Could you check a few things on this model? Use its own coordinates, in mm. A direction names the side the tool comes from. Give positions to 0.01 mm unless a question says otherwise; leave off trailing zeros. Loops run counter-clockwise (first coordinate to the right, second up) from the corner with the lowest first, then second, coordinate; pieces in that order, holes last. Notation, with made-up numbers: (17.5, 82.5) - (21.5, 82.5) arc R21 cw to (21.5, 111.5) - close; hole circle Ø11 at (-38, 73.25). An arc over 180 degrees is marked (long way). Write each question's results on one line, items separated by ' | '. Start each with the question number.
```python
from build123d import *

# Parameters (mm, degrees)
F2_R     = 30.5
F3_DEPTH = 2
F5_DEPTH = 2
F6_R     = 4.99999
F7_R     = 3


# Not quite as in the source:
# - a fillet or chamfer is up to 0.001 mm smaller than in the source, because OpenCascade refuses the exact size
# - a feature names something its author has since deleted; it is built from what else it names


with BuildPart() as f1:
    # F0 (on Top) → F1 (revolve)
    with BuildSketch(Plane.XY):
        Polygon((-22.6666666667, 22), (-22.6666666667, 17), (0, 17), (14.7224318643, 25.5), (31.7224318643, 25.5), (31.7224318643, 30.5), (13.3826859022, 30.5), (-1.3397459622, 22), align=None)
    revolve(axis=Axis((-8.7595172226, 0, 0), (1, 0, 0)))

    # F2 (on face) → F3 (join)
    with BuildSketch(Plane.YZ.offset(31.7224318643)):
        Circle(F2_R)
    extrude(amount=F3_DEPTH)

    # F4 (on face) → F5 (cut, through all)
    with BuildSketch(Plane.YZ.offset(33.7224318643)):
        with BuildLine():
            ThreePointArc((20.5, 15.1657508881), (18.1785168447, 17.8827158264), (15.5, 20.2484567313))
            Line((15.5, 20.2484567313), (15.5, -20.2484567313))
            ThreePointArc((15.5, -20.2484567313), (18.1785168447, -17.8827158264), (20.5, -15.1657508881))
            Line((20.5, -15.1657508881), (20.5, 15.1657508881))
        make_face()
        with BuildLine():
            ThreePointArc((14.5, 20.9761769634), (12.0750373532, 22.4598190758), (9.5, 23.6643191324))
            Line((9.5, 23.6643191324), (9.5, -23.6643191324))
            ThreePointArc((9.5, -23.6643191324), (12.0750373532, -22.4598190758), (14.5, -20.9761769634))
            Line((14.5, -20.9761769634), (14.5, 20.9761769634))
        make_face()
        with BuildLine():
            ThreePointArc((8.5, 24.0416305603), (6.0307786652, 24.7765959868), (3.5, 25.2586618806))
            Line((3.5, 25.2586618806), (3.5, -25.2586618806))
            ThreePointArc((3.5, -25.2586618806), (6.0307786652, -24.7765959868), (8.5, -24.0416305603))
            Line((8.5, -24.0416305603), (8.5, 24.0416305603))
        make_face()
        with BuildLine():
            ThreePointArc((2.5, 25.3771550809), (1.2515081776, 25.4692702542), (0, 25.5))
            ThreePointArc((0, 25.5), (-1.2515081776, 25.4692702542), (-2.5, 25.3771550809))
            Line((-2.5, 25.3771550809), (-2.5, -25.3771550809))
            ThreePointArc((-2.5, -25.3771550809), (-1.2515081776, -25.4692702542), (0, -25.5))
            ThreePointArc((0, -25.5), (1.2515081776, -25.4692702542), (2.5, -25.3771550809))
            Line((2.5, -25.3771550809), (2.5, 25.3771550809))
        make_face()
        with BuildLine():
            Line((-3.5, -25.2586618806), (-3.5, 25.2586618806))
            ThreePointArc((-3.5, 25.2586618806), (-6.0307786652, 24.7765959868), (-8.5, 24.0416305603))
            Line((-8.5, 24.0416305603), (-8.5, -24.0416305603))
            ThreePointArc((-8.5, -24.0416305603), (-6.0307786652, -24.7765959868), (-3.5, -25.2586618806))
        make_face()
        with BuildLine():
            Line((-9.5, -23.6643191324), (-9.5, 23.6643191324))
            ThreePointArc((-9.5, 23.6643191324), (-12.0750373532, 22.4598190758), (-14.5, 20.9761769634))
            Line((-14.5, 20.9761769634), (-14.5, -20.9761769634))
            ThreePointArc((-14.5, -20.9761769634), (-12.0750373532, -22.4598190758), (-9.5, -23.6643191324))
        make_face()
        with BuildLine():
            Line((-15.5, -20.2484567313), (-15.5, 20.2484567313))
            ThreePointArc((-15.5, 20.2484567313), (-18.1785168447, 17.8827158264), (-20.5, 15.1657508881))
            Line((-20.5, 15.1657508881), (-20.5, -15.1657508881))
            ThreePointArc((-20.5, -15.1657508881), (-18.1785168447, -17.8827158264), (-15.5, -20.2484567313))
        make_face()
        with BuildLine():
            Line((-21.5, -13.7113092008), (-21.5, 13.7113092008))
            ThreePointArc((-21.5, 13.7113092008), (-25.5, 0), (-21.5, -13.7113092008))
        make_face()
        with BuildLine():
            ThreePointArc((25.5, 0), (24.4795833298, 7.1414284285), (21.5, 13.7113092008))
            Line((21.5, 13.7113092008), (21.5, -13.7113092008))
            ThreePointArc((21.5, -13.7113092008), (24.4795833298, -7.1414284285), (25.5, 0))
        make_face()
    extrude(amount=-F5_DEPTH, mode=Mode.SUBTRACT)

    # F6 (radius 5 in the source; OpenCascade refuses exactly that, so slightly less here)
    f6_edges = [f1.edges().sort_by_distance(p)[0] for p in [
        (-22.666667, -22, 0),
        (-1.339746, -22, 0),
        (13.382686, -30.5, 0),
    ]]
    fillet(f6_edges, radius=F6_R)

    # F7
    f7_edges = [f1.edges().sort_by_distance(p)[0] for p in [
        (14.722432, -25.5, 0),
        (0, -17, 0),
    ]]
    fillet(f7_edges, radius=F7_R)


solid = f1.part
```
Q1. I want a section at A-A, the plane x = 21.5. List the corners of the cut face in (y, z) for me.
Q2. If we mould it in two halves opening along X, with no side actions, what happens to faces 4 (the face through (33, -8.5, 0)), 5 (the face through (1.53, -3.877, -17.458)), 6 (the face through (33.722, 9, 0))? For each: +X half, -X half, draft (parallel to the pull), parting line (faces both ways), or undercut.
Q3. I want a section at B-B, the plane z = -8. State how many separate pieces and enclosed holes the cut face has, then the cut area to 3 significant figures.
Q4. Which directions (+Z, -Z, +X, -X, +Y, -Y) give clear straight access to the entire face, cutting with the end or side of a thin tool? Please do faces 1 (the face through (24.089, -24.204, -18.559)), 2 (the face through (-10.28, 20.32, -8.43)), 3 (the face through (33, 3.5, 0)).
Q5. I want a section at D-D, the plane x = -8. List the corners of the cut face in (y, z) for me, then the cut area to 3 significant figures.
Q6. I'm going to push flat-ended pins straight in: pin 1 Ø12 at (x, z) = (-7, 21) entering from -Y; pin 2 Ø3 at (x, z) = (26.5, -7.5) entering from -Y; pin 3 Ø5 at (x, z) = (25.5, 2) entering from +Y; pin 4 Ø2 at (x, z) = (32.5, -4) entering from +Y. Where does each tip first touch, or does it pass through?
Q7. I need wall thicknesses on L1, parallel to Z at x = 26, y = 1; L2, parallel to Y at x = -10, z = 0.5; L3, parallel to Y at x = 19.5, z = 0. Which ranges of each line are inside material? Lowest first, please. Write a range as from..to.
Conclusion:
1) outline: circle Ø61 at (0, 0); hole circle Ø51 at (0, 0)
2) face 4: draft | face 5: undercut | face 6: +X half
3) separate pieces: 10 | enclosed holes: 0 | area: 633 mm^2
4) face 1: +X, -X | face 2: -X | face 3: +X
5) outline: circle Ø44 at (0, 0); hole circle Ø34 at (0, 0) | area: 613 mm^2
6) pin 1: y = -16.09 | pin 2: y = -29.9 | pin 3: y = 30.5 | pin 4: y = 30.35
7) L1: -30.48..-25.48, 25.48..30.48 | L2: -21.99..-16.99, 16.99..21.99 | L3: -30.5..-25.5, 25.5..30.5
